Can you work these out from the model? Positions are in its coordinate system, mm. Give positions to 0.01 mm unless a question says otherwise; leave off trailing zeros. Order: outer loops, then holes, each group sorted by start corner. A loop starts at its lowest first (then second) coordinate and runs counter-clockwise, first axis right, second up. Notation, with made-up numbers: (32.5, 31) - (65.5, 31) arc R14 ccw to (65.5, 50) - close; hole circle Ø10 at (5, 84.5). An arc over 180 degrees is marked (long way). One line per question, with ' | ' between items.
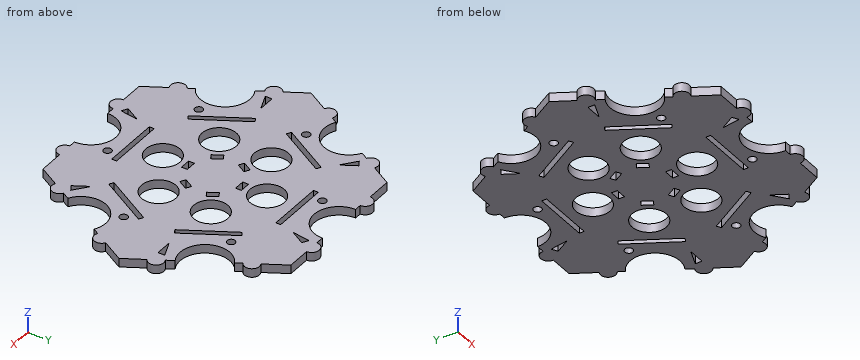
```python
from build123d import *

# Parameters (mm, degrees)
F0_R     = 6.992362
F0_W     = 22.860002
F0_H     = 1.970686
F0_W_2   = 4.335518
F0_H_2   = 2.364827
F1_DEPTH = 3.556
F2_R     = 1.625071
F3_DEPTH = 25.4


with BuildPart() as f1:
    # F0 (on Top) → F1 (new body)
    with BuildSketch(Plane.XY):
        with BuildLine():
            Line((-58.420235, 0), (0, 0))
            Line((0, 0), (-29.210117, 50.593407))
            Line((-29.210117, 50.593407), (-33.983866, 42.325032))
            ThreePointArc((-33.983866, 42.325032), (-38.230603, 41.187123), (-37.092693, 36.940386))
            Line((-37.092693, 36.940386), (-38.756345, 34.058855))
            ThreePointArc((-38.756345, 34.058855), (-35.053024, 20.237873), (-48.874007, 16.534552))
            Line((-48.874007, 16.534552), (-50.269638, 14.117248))
            ThreePointArc((-50.269638, 14.117248), (-54.441021, 12.999529), (-53.323302, 8.828147))
            Line((-53.323302, 8.828147), (-58.420235, 0))
        make_face()
        with Locations((-18.432006, 10.641724)):
            Circle(F0_R, mode=Mode.SUBTRACT)
        Polygon((-7.449457, 6.804059), (-9.617217, 3.04939), (-11.665217, 4.231803), (-9.497458, 7.986473), align=None, mode=Mode.SUBTRACT)
        Polygon((-33.875014, 6.35952), (-35.581678, 7.344863), (-24.151677, 27.142205), (-22.445013, 26.156862), align=None, mode=Mode.SUBTRACT)
        with BuildLine():
            Line((-29.210117, -50.593407), (0, 0))
            Line((0, 0), (-58.420235, 0))
            Line((-58.420235, 0), (-53.646486, -8.268375))
            ThreePointArc((-53.646486, -8.268375), (-54.784396, -12.515112), (-50.537659, -13.653022))
            Line((-50.537659, -13.653022), (-48.874007, -16.534552))
            ThreePointArc((-48.874007, -16.534552), (-35.053024, -20.237873), (-38.756345, -34.058855))
            Line((-38.756345, -34.058855), (-37.360714, -36.476159))
            ThreePointArc((-37.360714, -36.476159), (-38.478433, -40.647542), (-34.30705, -41.765261))
            Line((-34.30705, -41.765261), (-29.210117, -50.593407))
        make_face()
        Polygon((-22.445013, -26.156862), (-24.151677, -27.142205), (-35.581678, -7.344863), (-33.875014, -6.35952), align=None, mode=Mode.SUBTRACT)
        with Locations((-18.432006, -10.641724)):
            Circle(F0_R, mode=Mode.SUBTRACT)
        Polygon((-9.617217, -3.04939), (-7.449457, -6.804059), (-9.497458, -7.986473), (-11.665217, -4.231803), align=None, mode=Mode.SUBTRACT)
        with BuildLine():
            Line((-29.210117, 50.593407), (0, 0))
            Line((0, 0), (29.210117, 50.593407))
            Line((29.210117, 50.593407), (19.66262, 50.593407))
            ThreePointArc((19.66262, 50.593407), (16.553793, 53.702235), (13.444966, 50.593407))
            Line((13.444966, 50.593407), (10.117661, 50.593407))
            ThreePointArc((10.117661, 50.593407), (0, 40.475746), (-10.117661, 50.593407))
            Line((-10.117661, 50.593407), (-12.908924, 50.593407))
            ThreePointArc((-12.908924, 50.593407), (-15.962588, 53.647071), (-19.016252, 50.593407))
            Line((-19.016252, 50.593407), (-29.210117, 50.593407))
        make_face()
        with Locations((0, 33.501726)):
            Rectangle(F0_W, F0_H, mode=Mode.SUBTRACT)
        with Locations((0, 11.035863)):
            Rectangle(F0_W_2, F0_H_2, mode=Mode.SUBTRACT)
        with Locations((0, 21.283448)):
            Circle(F0_R, mode=Mode.SUBTRACT)
        with BuildLine():
            Line((29.210117, 50.593407), (0, 0))
            Line((0, 0), (58.420235, 0))
            Line((58.420235, 0), (53.646486, 8.268375))
            ThreePointArc((53.646486, 8.268375), (54.784396, 12.515112), (50.537659, 13.653022))
            Line((50.537659, 13.653022), (48.874007, 16.534552))
            ThreePointArc((48.874007, 16.534552), (35.053024, 20.237873), (38.756345, 34.058855))
            Line((38.756345, 34.058855), (37.360714, 36.476159))
            ThreePointArc((37.360714, 36.476159), (38.478433, 40.647542), (34.30705, 41.765261))
            Line((34.30705, 41.765261), (29.210117, 50.593407))
        make_face()
        Polygon((9.617217, 3.04939), (7.449457, 6.804059), (9.497458, 7.986473), (11.665217, 4.231803), align=None, mode=Mode.SUBTRACT)
        with Locations((18.432006, 10.641724)):
            Circle(F0_R, mode=Mode.SUBTRACT)
        Polygon((22.445013, 26.156862), (24.151677, 27.142205), (35.581678, 7.344863), (33.875014, 6.35952), align=None, mode=Mode.SUBTRACT)
        with BuildLine():
            Line((58.420235, 0), (0, 0))
            Line((0, 0), (29.210117, -50.593407))
            Line((29.210117, -50.593407), (33.983866, -42.325032))
            ThreePointArc((33.983866, -42.325032), (38.230603, -41.187123), (37.092693, -36.940386))
            Line((37.092693, -36.940386), (38.756345, -34.058855))
            ThreePointArc((38.756345, -34.058855), (35.053024, -20.237873), (48.874007, -16.534552))
            Line((48.874007, -16.534552), (50.269638, -14.117248))
            ThreePointArc((50.269638, -14.117248), (54.441021, -12.999529), (53.323302, -8.828147))
            Line((53.323302, -8.828147), (58.420235, 0))
        make_face()
        Polygon((33.875014, -6.35952), (35.581678, -7.344863), (24.151677, -27.142205), (22.445013, -26.156862), align=None, mode=Mode.SUBTRACT)
        Polygon((7.449457, -6.804059), (9.617217, -3.04939), (11.665217, -4.231803), (9.497458, -7.986473), align=None, mode=Mode.SUBTRACT)
        with Locations((18.432006, -10.641724)):
            Circle(F0_R, mode=Mode.SUBTRACT)
        with BuildLine():
            Line((29.210117, -50.593407), (0, 0))
            Line((0, 0), (-29.210117, -50.593407))
            Line((-29.210117, -50.593407), (-19.66262, -50.593407))
            ThreePointArc((-19.66262, -50.593407), (-16.553793, -53.702235), (-13.444966, -50.593407))
            Line((-13.444966, -50.593407), (-10.117661, -50.593407))
            ThreePointArc((-10.117661, -50.593407), (0, -40.475746), (10.117661, -50.593407))
            Line((10.117661, -50.593407), (12.908924, -50.593407))
            ThreePointArc((12.908924, -50.593407), (15.962588, -53.647071), (19.016252, -50.593407))
            Line((19.016252, -50.593407), (29.210117, -50.593407))
        make_face()
        with Locations((0, -33.501726)):
            Rectangle(F0_W, F0_H, mode=Mode.SUBTRACT)
        with Locations((0, -21.283448)):
            Circle(F0_R, mode=Mode.SUBTRACT)
        with Locations((0, -11.035863)):
            Rectangle(F0_W_2, F0_H_2, mode=Mode.SUBTRACT)
    extrude(amount=F1_DEPTH)

    # F2 (on face) → F3 (cut)
    with BuildSketch(Plane.XY.offset(3.556)):
        with Locations((8.079829, -38.428448)):
            Circle(F2_R)
        Polygon((-13.870498, -47.66334), (-12.809483, -40.399138), (-16.220229, -46.306723), align=None)
        Polygon((34.342414, -35.843874), (28.581938, -31.292907), (31.992684, -37.200492), align=None)
        with Locations((37.319927, -12.216887)):
            Circle(F2_R)
        Polygon((48.212913, 11.819466), (41.391421, 9.106231), (48.212913, 9.106231), align=None)
        with Locations((29.240098, 26.211561)):
            Circle(F2_R)
        Polygon((13.870498, 47.66334), (12.809483, 40.399138), (16.220229, 46.306723), align=None)
        with Locations((-8.079829, 38.428448)):
            Circle(F2_R)
        Polygon((-34.342414, 35.843874), (-28.581938, 31.292907), (-31.992684, 37.200492), align=None)
        with Locations((-37.319927, 12.216887)):
            Circle(F2_R)
        Polygon((-48.212913, -11.819466), (-41.391421, -9.106231), (-48.212913, -9.106231), align=None)
        with Locations((-29.240098, -26.211561)):
            Circle(F2_R)
    extrude(amount=-F3_DEPTH, mode=Mode.SUBTRACT)


solid = f1.part
```
(1) Will these pins go through, and if not, where does the flat tip stop? pin 1 (1.2 mm diameter, centred on y = -10.5, z = 2, fed in from +X); pin 2 (1.8 mm diameter, centred on x = 26.5, z = 1.5, fed in from -Y); pin 3 (2 mm diameter, centred on x = -32, y = -12.5, fed in from -Z); pin 4 (2 mm diameter, centred on y = -33.5, z = 2, fed in from +X).
Answer below:
pin 1: x = 54.83 | pin 2: y = -50.59 | pin 3: z = 0 | pin 4: x = 38.76
(2) Imagine slicing it at A-A (x = 0). List the corners of the cut face in (y, z) for me.
Answer below:
outline: (-40.48, 0) - (-34.49, 0) - (-34.49, 3.56) - (-40.48, 3.56) - close; (-32.52, 0) - (-28.28, 0) - (-28.28, 3.56) - (-32.52, 3.56) - close; (-14.29, 0) - (-12.22, 0) - (-12.22, 3.56) - (-14.29, 3.56) - close; (-9.85, 0) - (9.85, 0) - (9.85, 3.56) - (-9.85, 3.56) - close; (12.22, 0) - (14.29, 0) - (14.29, 3.56) - (12.22, 3.56) - close; (28.28, 0) - (32.52, 0) - (32.52, 3.56) - (28.28, 3.56) - close; (34.49, 0) - (40.48, 0) - (40.48, 3.56) - (34.49, 3.56) - close
(3) Imagine slicing it at B-B (z = 2.25). Count the separate pieces of the cut face and the enclosed holes in it, and give its area (3 significant figures).
Answer below:
separate pieces: 1 | enclosed holes: 30 | area: 6,720 mm^2
(4) If I drill on line 1 (Y direction, x = -9, z = 2.6); line 2 (Y direction, x = -6, z = 2.75); line 3 (Y direction, x = -35, z = 0.35), over which ranges is the centre line in solid material (lowest first)?
Answer below:
line 1: -45.97 to -34.49, -32.52 to -7.7, -4.12 to 4.12, 7.7 to 32.52, 34.49 to 37.09, 39.77 to 45.97 | line 2: -42.45 to -34.49, -32.52 to -24.87, -17.69 to 17.69, 24.87 to 32.52, 34.49 to 42.45 | line 3: -42.06 to -30.26, -20.33 to -8.35, -7.01 to 7.01, 8.35 to 20.33, 30.26 to 42.69
